Design review of the part built by this model. Coordinates are the model's own, in mm. Give positions to 0.01 mm unless a question says otherwise; leave off trailing zeros. Write each loop counter-clockwise with the first axis right and the second up, starting at its lowest first coordinate (ties: lowest second). Pieces come first, ordered by that corner, then holes. Notation, with made-up numbers: (7, -5.75) - (11, -5.75) arc R21 ccw to (11, 32.25) - close; hole circle Ø8 at (71.25, 81.25). An arc over 180 degrees is marked (long way). Use a Markdown table: item, result. Add a question column.
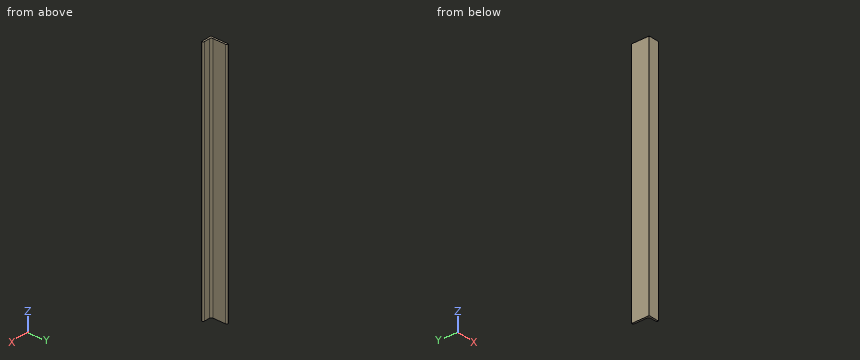
Autodesk Inventor part; units mm, degrees
ref_plane "Start Plane" through (0, 0, -100) normal (0, 0, 1) x (1, 0, 0)
ref_plane "End Plane" through (0, 0, 600) normal (0, 0, 1) x (1, 0, 0)
ref_plane "YZ Plane" through (0, 0, 0) normal (1, 0, 0) x (0, 1, 0)
ref_plane "Start Plane" through (0, 0, -100) normal (0, 0, 1) x (1, 0, 0)
ref_plane "End Plane" through (0, 0, 600) normal (0, 0, 1) x (1, 0, 0)
sketch "Sketch" plane through (0, 0, 0) normal (0, 0, 1) x (1, 0, 0)
  line L0 (-2.41, 28.7) -> (-2.41, -7.3)
  line L1 (-7.41, 32.7) -> (-6.41, 32.7)
  line L2 (-7.41, -17.3) -> (-7.41, 32.7)
  line L3 (22.59, -17.3) -> (-7.41, -17.3)
  line L4 (22.59, -16.3) -> (22.59, -17.3)
  line L5 (2.59, -12.3) -> (18.59, -12.3)
  arc A0 (-2.41, -7.3) -> (2.59, -12.3) centre (2.59, -7.3) ccw
  arc A1 (-2.41, 28.7) -> (-6.41, 32.7) centre (-6.41, 28.7) ccw
  arc A2 (22.59, -16.3) -> (18.59, -12.3) centre (18.59, -16.3) ccw
  line L6 (0, 43.6941) -> (0, -27.4657) construction
  line L7 (-13.5757, 0) -> (29.5841, 0) construction
  point P0 (-2.41, 32.7)
  point P1 (-2.41, -12.3)
  point P2 (22.59, -12.3)
  dimension "d4" = 30
  dimension "d6" = 50
  dimension "d8" = 5
  dimension "d10" = 5
  dimension "d17" = 5
  dimension "d18" = 4
  dimension "d19" = 17.3
  dimension "d20" = 7.41
extrude "Body" add sketch "Sketch" along normal up to surface (700 mm away) from surface at -100
sketch "Sketch3" plane through (0, 0, 0) normal (0, 0, 1) x (1, 0, 0)
  line L0 (0, 0) -> (10, 0)
ref_plane "Work Plane10" through (0, 0, 0) normal (0, -1, 0) x (1, 0, 0)
sketch "Sketch4" plane through (0, 0, 0) normal (0, -1, 0) x (1, 0, 0)
  line L0 (-2, -100) -> (12, -100)
  line L1 (-2, 600) -> (12, 600)
  dimension "d24" = 700
equation "\"d4\" = b"
equation "\"d6\" = ParH"
equation "\"d17\" = R"
equation "\"d18\" = R1"
equation "\"d19\" = ex"
equation "\"d20\" = ey"
equation "\"d11\" = G_L"
equation "\"b\" = 30"
equation "\"ParT\" = 5"
equation "\"R1\" = 4"
equation "\"G_L\" = d24"
equation "\"ParH\" = 50"
equation "\"R\" = 5"
equation "\"ey\" = 7.41"
equation "\"ex\" = 17.3"
equation "\"G_OFFSET_END\" = 0"
properties part number "ISO 657-2 - 50x 30x 5-700" material "Steel, Mild"
(1) Add section A-A (z = 237). State the section outline as (x, y) points, and give its area (3 significant figures).
(2) For line 1 along X through (y, z) = (24.5, 539.5); line 2 along Y through (x, z) = (6.75, 182); line 3 along X through (y, z) = (-11, 61.5), list the stretches that pass through material, from the lowest coordinate up.
(3) Add section B-B (x = 10.25). State the section outline as (y, z) points, and give its area (3 significant figures).
(4) Insertion check: pin 1 (10 mm diameter, centred on x = 7.5, y = 20.5, fed in from -Z); pin 2 (8 mm diameter, centred on x = 15, z = 350, fed in from +Y); pin 3 (3 mm diameter, centred on y = 24, z = 81.5, fed in from +X); pin 4 (1 mm diameter, centred on x = 1.5, z = 5, fed in from +Y). Each pin has a flat end and moves straight along its axis. Give the tip position at first contact, or say it passes through.
(5) Add section C-C (y = 5). State the section outline as (x, z) points.
Answers follow:
| question | item | result |
|---|---|---|
| 1 | outline | (-7.41, -17.3) - (22.59, -17.3) - (22.59, -16.3) arc R4 ccw to (18.59, -12.3) - (2.59, -12.3) arc R5 cw to (-2.41, -7.3) - (-2.41, 28.7) arc R4 ccw to (-6.41, 32.7) - (-7.41, 32.7) - close |
| 1 | area | 373 mm^2 |
| 2 | line 1 | -7.41 to -2.41 |
| 2 | line 2 | -17.3 to -12.3 |
| 2 | line 3 | -7.41 to -0.77 |
| 3 | outline | (-17.3, -100) - (-12.3, -100) - (-12.3, 600) - (-17.3, 600) - close |
| 3 | area | 3,500 mm^2 |
| 4 | pin 1 | through |
| 4 | pin 2 | y = -12.3 |
| 4 | pin 3 | x = -2.41 |
| 4 | pin 4 | y = -12.04 |
| 5 | outline | (-7.41, -100) - (-2.41, -100) - (-2.41, 600) - (-7.41, 600) - close |
